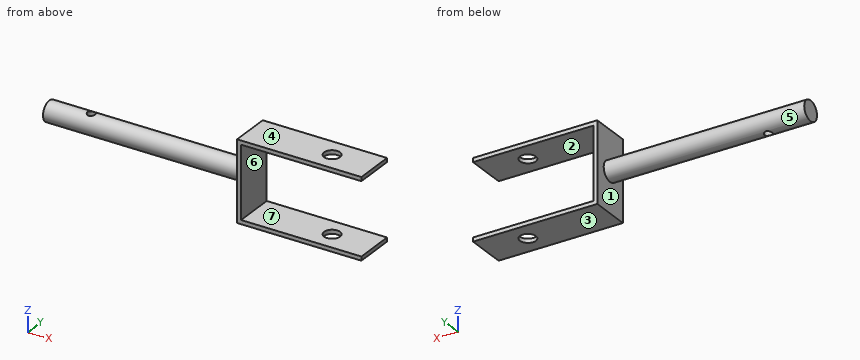
Autodesk Inventor part; units mm, degrees
ref_plane "YZ Plane" through (0, 0, 0) normal (1, 0, 0) x (0, 1, 0)
ref_plane "XZ Plane" through (0, 0, 0) normal (0, 1, 0) x (-1, 0, 0)
ref_plane "XY Plane" through (0, 0, 0) normal (0, 0, 1) x (1, 0, 0)
sketch "草图1" plane through (0, 0, 0) normal (1, 0, 0) x (0, 1, 0)
  circle A0 centre (0, 0) radius 2.5
  dimension "杆直径" = 5
extrude "拉伸1" add sketch "草图1" along normal blind 50
sketch "草图2" plane through (50, 0, 0) normal (1, 0, 0) x (0, 0, -1)
  line L0 (10, -5) -> (-10, -5)
  line L1 (-10, -5) -> (-10, 5)
  line L2 (-10, 5) -> (10, 5)
  line L3 (10, 5) -> (10, -5)
  line L4 (10, -5) -> (-10, 5) construction
  line L5 (-10, -5) -> (10, 5) construction
  point P0 (0, 0)
  dimension "框长" = 20
  dimension "框宽" = 10
extrude "拉伸2" add sketch "草图2" along normal blind 1
sketch "草图3" plane through (51, 0, 0) normal (1, 0, 0) x (0, 0, -1)
  line L0 (-10, -5) -> (10, -5)
  line L1 (10, -5) -> (10, 5)
  line L2 (10, 5) -> (-10, 5)
  line L3 (-10, 5) -> (-10, -5)
  line L4 (-10, 5) -> (-9, 5)
  line L5 (-9, 5) -> (-9, -5)
  line L6 (10, 5) -> (9, 5)
  line L7 (9, 5) -> (9, -5)
  point P0 (0, 0)
  dimension "d7" = 1
  dimension "d8" = 1
extrude "拉伸3" add sketch "草图3" along normal blind 30 contours L3 L2 L5 L0 | L7 L2 L1 L0
hole "孔1" at (70.5, 0, -10) direction (0, 0, 1) diameter 4 end through all
sketch "草图5" plane through (0, 0, 0) normal (0, 0, 1) x (1, 0, 0)
  circle A0 centre (70.5, 0) radius 2
  line L0 (50, -2.5) -> (50, 2.5)
  line L1 (0, 2.5) -> (0, -2.5)
  line L2 (70.5, 0) -> (10.5, 0)
  circle A1 centre (10.5, 0) radius 1
  point P0 (0, 0)
  dimension "高度" = 60
  dimension "销孔径" = 2
extrude "拉伸4" cut sketch "草图5" along normal mid plane 10 contours A1
properties part number "顶杆" material "木材(桦木)"
Verification items for the finished model (mm, model axes). Face numbers are marked on the shaded views. A direction names the side the tool comes from. Coordinates: 2 decimals unless noted, no trailing zeros. Loops run counter-clockwise (first coordinate to the right, second up) from the corner with the lowest first, then second, coordinate; pieces in that order, holes last. Notation, with made-up numbers: (50, 61) - (90, 61) arc R13 cw to (90, 69) - close; hole circle Ø10 at (41, -31.5). An arc over 180 degrees is marked (long way). Answer as a JSON object with one key per item and string values.
(1) Scan lines: line 1 along X through (y, z) = (0, 9.85); line 2 along Z through (x, y) = (53, 2); line 3 along Y through (x, z) = (70.5, -9.6). Record each from-to range of solid material in increasing order.
Response:
{"line 1": "x = 50 to 68.5, 72.5 to 81", "line 2": "z = -10 to -9, 9 to 10", "line 3": "y = -5 to -2, 2 to 5"}
(2) Cross-section at D-D, the plane x = 13. Record the boundary of the cut face in (y, z), then the cut area to 3 significant figures.
Response:
{"outline": "circle Ø5 at (0, 0)", "area": "19.6 mm²"}
(3) Cross-section at B-B, the plane z = 0. Record the boundary of the cut face in (x, y), then the cut area to 3 significant figures.
Response:
{"outline": "(0, -2.5) - (50, -2.5) - (50, -5) - (51, -5) - (51, 5) - (50, 5) - (50, 2.5) - (0, 2.5) - close; hole circle Ø2 at (10.5, 0)", "area": "257 mm²"}
(4) Cross-section at A-A, the plane x = 70.5. Record the boundary of the cut face in (y, z), then the cut area to 3 significant figures.
Response:
{"outline": "(-5, -10) - (-2, -10) - (-2, -9) - (-5, -9) - close; (-5, 9) - (-2, 9) - (-2, 10) - (-5, 10) - close; (2, -10) - (5, -10) - (5, -9) - (2, -9) - close; (2, 9) - (5, 9) - (5, 10) - (2, 10) - close", "area": "12.0 mm²"}
(5) Access from +Z, -Z, +X, -X, +Y, -Y to the whole of each face (thin tool, end or side, straight path). Record for the marked faces 1, 2 and 3.
Response:
{"face 1": "-X", "face 2": "+X, +Y, -Y", "face 3": "-Z, +X, -X, +Y, -Y"}
(6) Go/stop test with flat-tipped pins: pin 1 Ø2 at (x, y) = (13, 1.5) entering from +Z; pin 2 Ø1.5 at (y, z) = (-3.5, -4) entering from +X; pin 3 Ø3 at (x, y) = (10.5, 0) entering from -Z. Record where each tip stops, or that it passes through.
Response:
{"pin 1": "stops at z = 2.45", "pin 2": "stops at x = 51", "pin 3": "stops at z = -2.5"}
(7) Mould release check, pull along Z, two halves, no side actions. Record for the marked faces 4, 5, 6 and 7: pulls with the +Z half, pulls with the -Z half, needs draft (parallel to the pull), parting line crosses it, or undercut.
Response:
{"face 4": "pulls with the +Z half", "face 5": "parting line crosses it", "face 6": "undercut", "face 7": "undercut"}
(8) Cross-section at C-C, the plane x = 60.5. Record the boundary of the cut face in (y, z), then the cut area to 3 significant figures.
Response:
{"outline": "(-5, -10) - (5, -10) - (5, -9) - (-5, -9) - close; (-5, 9) - (5, 9) - (5, 10) - (-5, 10) - close", "area": "20.0 mm²"}
